```python
from build123d import *

# Parameters (mm, degrees)
SKETCH1_W           = 292
SKETCH1_H           = 107
BOSS_EXTRUDE1_DEPTH = 3
SKETCH8_W           = 3
SKETCH8_H           = 35
CUT_EXTRUDE7_DEPTH  = 3
SKETCH7_W           = 35
SKETCH7_H           = 3
BOSS_EXTRUDE2_DEPTH = 3
SKETCH4_W           = 35
SKETCH4_H           = 3
BOSS_EXTRUDE3_DEPTH = 3
SKETCH9_R           = 1.5
CUT_EXTRUDE8_DEPTH  = 10


with BuildPart() as part:
    # Sketch1 → Boss-Extrude1 (new body)
    with BuildSketch(Plane(origin=(0, 0, 0), x_dir=(1, 0, 0), z_dir=(0, 1, 0))):
        Rectangle(SKETCH1_W, SKETCH1_H)
    extrude(amount=BOSS_EXTRUDE1_DEPTH)

    # Sketch8 → Cut-Extrude7 (cut)
    with BuildSketch(Plane(origin=(0, 3, 0), x_dir=(1, 0, 0), z_dir=(0, 1, 0))):
        with Locations((144.5, 0)):
            Rectangle(SKETCH8_W, SKETCH8_H)
        with Locations((-144.5, 0)):
            Rectangle(SKETCH8_W, SKETCH8_H)
    extrude(amount=-CUT_EXTRUDE7_DEPTH, mode=Mode.SUBTRACT)

    # Sketch7 → Boss-Extrude2 (add)
    with BuildSketch(Plane(origin=(0, 3, 0), x_dir=(1, 0, 0), z_dir=(0, 1, 0))):
        with Locations((0, -55)):
            Rectangle(SKETCH7_W, SKETCH7_H)
        with Locations((0, 55)):
            Rectangle(SKETCH7_W, SKETCH7_H)
    extrude(amount=-BOSS_EXTRUDE2_DEPTH)

    # Sketch4 → Boss-Extrude3 (add)
    with BuildSketch(Plane(origin=(0, 3, 0), x_dir=(1, 0, 0), z_dir=(0, 1, 0))):
        with Locations((-103.5, -55)):
            Rectangle(SKETCH4_W, SKETCH4_H)
        with Locations((-103.5, 55)):
            Rectangle(SKETCH4_W, SKETCH4_H)
        with Locations((103.5, 55)):
            Rectangle(SKETCH4_W, SKETCH4_H)
        with Locations((103.5, -55)):
            Rectangle(SKETCH4_W, SKETCH4_H)
    extrude(amount=-BOSS_EXTRUDE3_DEPTH)

    # Sketch9 → Cut-Extrude8 (cut)
    with BuildSketch(Plane(origin=(0, 3, 0), x_dir=(1, 0, 0), z_dir=(0, 1, 0))):
        with Locations(Location((-27.565814615, -37.860553904, 0), (0, 0, 270))):
            Circle(SKETCH9_R)
        with Locations(Location((-51.565814615, -37.860553904, 0), (0, 0, 270))):
            Circle(SKETCH9_R)
        with BuildLine():
            Line((-42.765814615, -36.560553904), (-36.365814615, -36.560553904))
            ThreePointArc((-36.365814615, -36.560553904), (-35.065814615, -37.860553904), (-36.365814615, -39.160553904))
            Line((-36.365814615, -39.160553904), (-42.765814615, -39.160553904))
            ThreePointArc((-42.765814615, -39.160553904), (-44.065814615, -37.860553904), (-42.765814615, -36.560553904))
        make_face()
    extrude(amount=-CUT_EXTRUDE8_DEPTH, mode=Mode.SUBTRACT)


solid = part.part
```
The model under review builds one solid part; all positions refer to its coordinate system, in mm. Give positions to 0.01 mm unless a question says otherwise; leave off trailing zeros. Write each loop counter-clockwise with the first axis right and the second up, starting at its lowest first coordinate (ties: lowest second). Pieces come first, ordered by that corner, then holes. Notation, with made-up numbers: (86.5, 59) -> (145.5, 59) arc R30 ccw to (145.5, 98) -> close; hole circle Ø8 at (12.5, 65). An arc over 180 degrees is marked (long way). Answer in a Markdown table with one row per item.
1) Add section B-B on y = 2.1. Count the separate pieces of the cut face and the enclosed holes in it, plus the area to 3 significant figures.
Worked answers:
| item | result |
|---|---|
| separate pieces | 1 |
| enclosed holes | 3 |
| area | 31,600 mm² |
2) For L1, parallel to Z at x = -61, y = 2; L2, parallel to X at y = 1.35, z = 0.5, list the stretches that pass through material, from the lowest coordinate up. Write a range as [from, to].
Worked answers:
| item | result |
|---|---|
| L1 | [-53.5, 53.5] |
| L2 | [-143, 143] |
3) Clearance check with flat-ended pins moving along their axes: P1, Ø1.5, axis at y = 1.5, z = -55, coming from the +X side; P2, Ø0.9, axis at x = 39.5, y = 1.5, coming from the -Z side; P3, Ø1.5, axis at y = 1.5, z = -11, coming from the -X side. State where each tip first meets the part, or that it passes through.
Worked answers:
| item | result |
|---|---|
| P1 | x = 121 |
| P2 | z = -53.5 |
| P3 | x = -143 |
4) Add section A-A on x = 62.5. State the section outline as (y, z) points.
Worked answers:
| item | result |
|---|---|
| outline | (0, -53.5) -> (3, -53.5) -> (3, 53.5) -> (0, 53.5) -> close |
